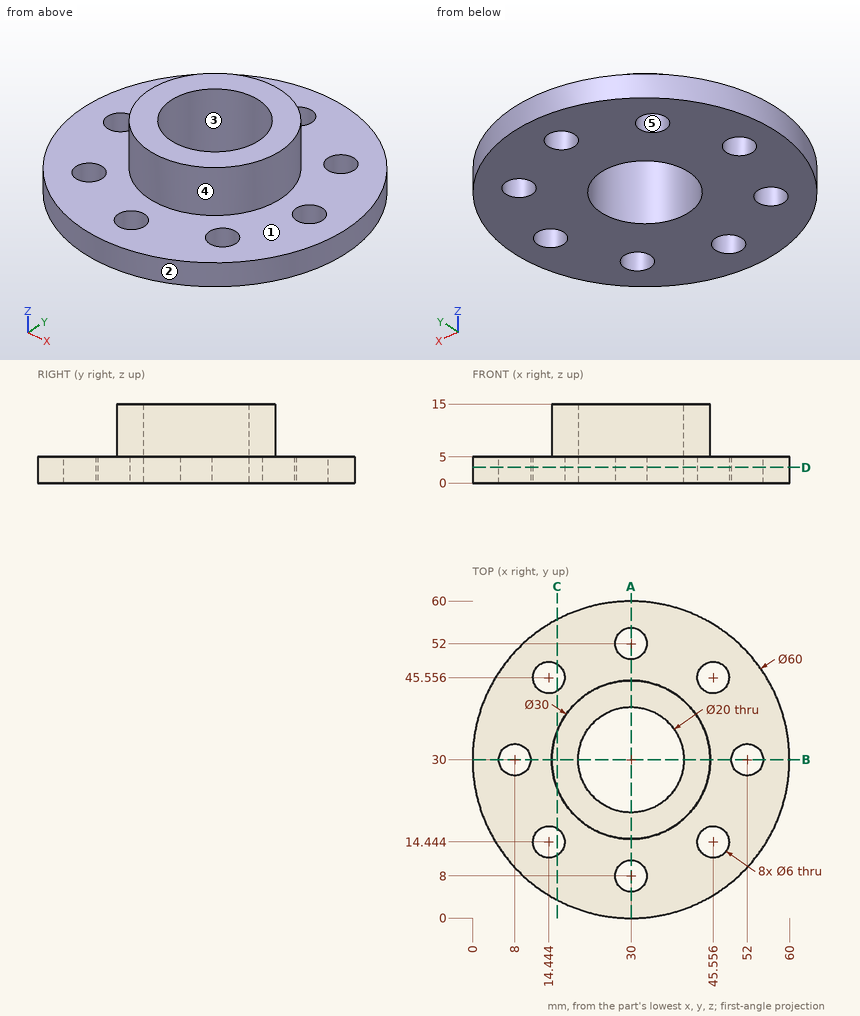
Source: three-view drawing plus pictorial views. Frame: mm from the lowest corner of the part. A direction names the side the tool comes from. Coordinates: 2 decimals unless noted, no trailing zeros. Write each loop counter-clockwise with the first axis right and the second up, starting at its lowest first coordinate (ties: lowest second). Pieces come first, ordered by that corner, then holes. Notation, with made-up numbers: (70, 54.25) - (99, 54.25) arc R27 ccw to (99, 73.25) - close; hole circle Ø2 at (-36.5, -6). An arc over 180 degrees is marked (long way). Answer as a JSON object with one key per item and string values.
Q1. Material intervals for line 1 (Y direction, x = 16.5, z = 3.5); line 2 (Z direction, x = 11, y = 46.5); line 3 (Y direction, x = 30, z = 8), sorted ascending. Write a range as [from, to].
Ans:
{"line 1": "y = [3.21, 12.26], [16.63, 43.37], [47.74, 56.79]", "line 2": "z = [0, 5]", "line 3": "y = [15, 20], [40, 45]"}
Q2. Draft query along Y for the marked faces 1, 2 and 3. Return one class per face: released by +Y, released by -Y, zero draft, split by the parting line, or undercut.
Ans:
{"face 1": "zero draft", "face 2": "split by the parting line", "face 3": "undercut"}
Q3. First-contact query: pin 1 Ø7 at (x, y) = (45.56, 45.56) entering from +Z; pin 2 Ø5 at (x, z) = (25.5, 13) entering from +Y; pin 3 Ø1.5 at (x, z) = (19, 10) entering from +Y. Flat tips, straight axial feed; report the tip coordinate or a pass-through.
Ans:
{"pin 1": "stops at z = 5", "pin 2": "stops at y = 44.87", "pin 3": "stops at y = 40.95"}
Q4. Section query D-D, the plane z = 3. State how many separate pieces and enclosed holes the cut face has, plus the area to 3 significant figures.
Ans:
{"separate pieces": "1", "enclosed holes": "9", "area": "2,290 mm2"}
Q5. Set-up query: the marked faces 4 and 5. Return all of +Z, -Z, +X, -X, +Y, -Y with unobstructed straight access to the full face (end or side cutting, diameter ignored); none if empty.
Ans:
{"face 4": "+Z", "face 5": "+Z, -Z"}
Q6. Section query A-A, the plane x = 30. Output: boundary loops of the cut face in (y, z).
Ans:
{"outline": "(0, 0) - (5, 0) - (5, 5) - (0, 5) - close; (11, 0) - (20, 0) - (20, 15) - (15, 15) - (15, 5) - (11, 5) - close; (40, 0) - (49, 0) - (49, 5) - (45, 5) - (45, 15) - (40, 15) - close; (55, 0) - (60, 0) - (60, 5) - (55, 5) - close"}
Q7. Section query C-C, the plane x = 16. Output: boundary loops of the cut face in (y, z) (1 decimal), plus the area to 3 significant figures.
Ans:
{"outline": "(3.5, 0) - (11.9, 0) - (11.9, 5) - (3.5, 5) - close; (17, 0) - (43, 0) - (43, 5) - (35.4, 5) - (35.4, 15) - (24.6, 15) - (24.6, 5) - (17, 5) - close; (48.1, 0) - (56.5, 0) - (56.5, 5) - (48.1, 5) - close", "area": "322 mm2"}
